Part model, mm, in its own coordinate system. Face numbers are marked on the shaded views. A direction names the side the tool comes from. Coordinates: 2 decimals unless noted, no trailing zeros. Write each loop counter-clockwise with the first axis right and the second up, starting at its lowest first coordinate (ties: lowest second). Pieces come first, ordered by that corner, then holes. Notation, with made-up numbers: (55, 78.25) -> (114, 78.25) arc R19 cw to (114, 89.25) -> close; hole circle Ø7 at (68, 69.5). An arc over 180 degrees is marked (long way). Write item = value, one per line.
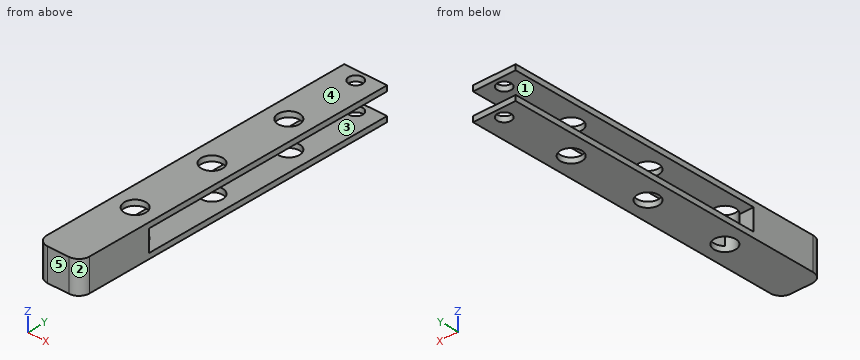
from build123d import *

# Parameters (mm, degrees)
F0_R     = 6.35
F0_R_2   = 4.136422
F1_DEPTH = 19.05
F2_W     = 12.7
F2_H     = 12.7
F3_DEPTH = 152.4


with BuildPart() as f1:
    # F0 (on Top) → F1 (new body)
    with BuildSketch(Plane.XY):
        with BuildLine():
            Line((25.4, 6.35), (25.4, 196.85))
            Line((25.4, 196.85), (6.35, 196.85))
            Line((6.35, 196.85), (0, 196.85))
            Line((0, 196.85), (0, 190.5))
            Line((0, 190.5), (0, 98.425))
            Line((0, 98.425), (0, 6.35))
            ThreePointArc((0, 6.35), (1.859872, 1.859872), (6.35, 0))
            Line((6.35, 0), (19.05, 0))
            ThreePointArc((19.05, 0), (23.540128, 1.859872), (25.4, 6.35))
        make_face()
        with Locations((12.7, 49.2125)):
            Circle(F0_R, mode=Mode.SUBTRACT)
        with Locations((12.7, 98.425)):
            Circle(F0_R, mode=Mode.SUBTRACT)
        with Locations((12.7, 147.6375)):
            Circle(F0_R, mode=Mode.SUBTRACT)
        with Locations((12.7, 190.5)):
            Circle(F0_R_2, mode=Mode.SUBTRACT)
    extrude(amount=F1_DEPTH)

    # F2 (on face) → F3 (cut)
    with BuildSketch(Plane(origin=(0, 196.85, 0), x_dir=(-1, 0, 0), z_dir=(0, 1, 0))):
        with Locations((-19.05, 9.525)):
            Rectangle(F2_W, F2_H)
        with Locations((-6.35, 9.525)):
            Rectangle(F2_W, F2_H)
    extrude(amount=-F3_DEPTH, mode=Mode.SUBTRACT)


solid = f1.part
Q1. Mould opens along Z. For the marked faces 3, 4 and 5 say: released by +Z, released by -Z, zero draft, split by the parting line, or undercut.
Model answer:
face_3 = undercut
face_4 = released by +Z
face_5 = zero draft
Q2. Saw through at B-B on y = 87.5. Give the cut face in (x, z) (3 decimals), and give its area (3 significant figures).
Model answer:
outline = (0, 0) -> (25.4, 0) -> (25.4, 3.175) -> (0, 3.175) -> close; (0, 15.875) -> (25.4, 15.875) -> (25.4, 19.05) -> (0, 19.05) -> close
area = 161 mm²
Q3. Pin check, flat tip, straight feed: pin 1 (4 mm diameter, centred on x = 20.5, z = 9.5, fed in from +Y). Stop position of the tip, or through.
Model answer:
pin_1 = 44.45
Q4. Which spindle directions (+Z, -Z, +X, -X, +Y, -Y) get a long thin tool onto all of the face, cutting with end or side? Do the marked faces 1 and 2. Say none if no direction does.
Model answer:
face_1 = +X, -X, +Y
face_2 = +Z, -Z, +X, -Y
Q5. Saw through at D-D on x = 12.7. Count the separate pieces of the cut face and the enclosed holes in it, and give its area (3 significant figures).
Model answer:
separate_pieces = 9
enclosed_holes = 0
area = 1,500 mm²
Q6. Probe line 1 (Z direction, x = 5.5, y = 93) (3 decimals); line 2 (Y direction, x = 17.25, z = 16.5); line 3 (Y direction, x = 19.5, z = 17.25). List the from-to ranges inside material, lowest first. Write a range as from..to.
Model answer:
line_1 = 0..3.175, 15.875..19.05
line_2 = 0..44.78, 53.64..94, 102.85..143.21, 152.07..196.85
line_3 = 0.02..196.85
Q7. Saw through at C-C on z = 12.5. Give the cut face in (x, y).
Model answer:
outline = (0, 6.35) arc R6.35 ccw to (6.35, 0) -> (19.05, 0) arc R6.35 ccw to (25.4, 6.35) -> (25.4, 44.45) -> (16.9, 44.45) arc R6.35 cw to (8.5, 44.45) -> (0, 44.45) -> close
Q8. Saw through at A-A on y = 190.5. Give the cut face in (x, z) (3 decimals), and give its area (3 significant figures).
Model answer:
outline = (0, 0) -> (8.564, 0) -> (8.564, 3.175) -> (0, 3.175) -> close; (0, 15.875) -> (8.564, 15.875) -> (8.564, 19.05) -> (0, 19.05) -> close; (16.836, 0) -> (25.4, 0) -> (25.4, 3.175) -> (16.836, 3.175) -> close; (16.836, 15.875) -> (25.4, 15.875) -> (25.4, 19.05) -> (16.836, 19.05) -> close
area = 109 mm²
